```python
from build123d import *

# Parameters (mm, degrees)
SKETCH1_R          = 2.6924
EXTRUDE3_DEPTH     = 1.2446
SKETCH4_W          = 15.875
SKETCH4_H          = 1.4224
CHAMFER1_SIZE      = 0.47625
SKETCH26_R         = 0.7112
EXTRUDE8_DEPTH     = 1.2446
CUT_EXTRUDE3_REACH = 18.325
CIRPATTERN1_COUNT  = 4
DRAFT2_ANGLE       = 5


# Read off the part's stored shape, not the designer's step: Extrude10, Draft1
with BuildPart() as part:
    # Sketch1 → Extrude3 (new body)
    with BuildSketch(Plane.XY):
        Circle(SKETCH1_R)
    extrude(amount=EXTRUDE3_DEPTH)

    # Sketch11 → Cut-Revolve3 (revolve, cut)
    with BuildSketch(Plane(origin=(0, 0, 0), x_dir=(0, 0, -1), z_dir=(1, 0, 0)), mode=Mode.PRIVATE) as cut_revolve3_sk:
        Polygon((0, 1.209143479), (-1.2446, 2.6924), (0, 2.6924), align=None)
    revolve(cut_revolve3_sk.sketch.rotate(Axis((0, 0, -0.441444004), (0, 0, 1)), 90), axis=Axis((0, 0, -0.441444004), (0, 0, 1)), mode=Mode.SUBTRACT)

    # Extrude10 outline → Extrude10 (revolve)
    with BuildSketch(Plane.XZ):
        Polygon((1.4224, 0), (1.4224, 0.178943468), (1.209143479, 0.178943468), (1.209143479, 0), (0, 0), (0, -1.4224), align=None)
    revolve(axis=Axis((0, 0, 0), (0, 0, 1)))



with BuildPart() as body_2:
    # Sketch4 → Revolve1 (revolve)
    with BuildSketch(Plane(origin=(0, 0, 0), x_dir=(0, 0, -1), z_dir=(1, 0, 0)), mode=Mode.PRIVATE) as revolve1_sk:
        with Locations((6.6929, 0.7112)):
            Rectangle(SKETCH4_W, SKETCH4_H)
    revolve(revolve1_sk.sketch.rotate(Axis((0, 0, 1.2446), (0, 0, -1)), 180), axis=Axis((0, 0, 1.2446), (0, 0, -1)))

    # Chamfer1
    chamfer1_edges = [body_2.edges().sort_by_distance(p)[0] for p in [
        (0, 1.4224, -14.6304),
    ]]
    chamfer(chamfer1_edges, length=CHAMFER1_SIZE)


with BuildPart() as part_1:
    add(part.part)

    add(body_2.part)  # Extrude8 merges body 2
    # Sketch26 → Extrude8 (add)
    with BuildSketch(Plane.XY.offset(1.2446)):
        Circle(SKETCH26_R)
    extrude(amount=-EXTRUDE8_DEPTH)

    # Cut-Extrude3: up to this cone (the profile starts inside it)
    cut_extrude3_end = Plane(origin=(0, 0, 1.2446), z_dir=(0, 0, 1)).offset(-1.673411083) * Cone(1.192e-06, 26.805764308, 22.492705944, align=(Align.CENTER, Align.CENTER, Align.MIN), mode=Mode.PRIVATE)
    # Sketch12 → Cut-Extrude3 (cut, up to the surface)
    with BuildSketch(Plane.XY.offset(1.2446), mode=Mode.PRIVATE) as cut_extrude3_sk1:
        with BuildLine():
            Line((1.758668316, 0.358986667), (1.058827491, 0.358986667))
            Line((1.058827491, 0.358986667), (0.563965298, 0.563965298))
            Line((0.563965298, 0.563965298), (0.358986667, 1.058827491))
            Line((0.358986667, 1.058827491), (0.358986667, 1.758668316))
            ThreePointArc((0.358986667, 1.758668316), (0.180406886, 1.785844066), (0, 1.794933333))
            Line((0, 1.794933333), (0, 0))
            Line((0, 0), (1.794933333, 0))
            ThreePointArc((1.794933333, 0), (1.785844066, 0.180406886), (1.758668316, 0.358986667))
        make_face()
    cut_extrude3_tool1 = extrude(cut_extrude3_sk1.sketch, amount=-CUT_EXTRUDE3_REACH, mode=Mode.PRIVATE) & cut_extrude3_end
    cut_extrude3 = cut_extrude3_tool1.solids().sort_by_distance((1.408748, 0.333602, 1.2446))[0]
    add(cut_extrude3, mode=Mode.SUBTRACT)

    # CirPattern1: Cut-Extrude3 ×4 about axis
    cirpattern1_axis = Axis((0, 0, 0), (0, 0, 1))
    for i in range(1, CIRPATTERN1_COUNT):
        add(cut_extrude3.rotate(cirpattern1_axis, i * 360 / CIRPATTERN1_COUNT), mode=Mode.SUBTRACT)

    # Draft1 outline → Draft1 (revolve)
    with BuildSketch(Plane.XZ):
        Polygon((1.794933333, 1.2446), (1.737108581, 1.028795087), (1.794933333, 1.028795087), align=None)
    revolve(axis=Axis((0, 0, 0), (0, 0, 1)))

    # Draft2
    draft2_faces = [part_1.faces().sort_by_distance(p)[0] for p in [
        (0.358986667, 1.329150829, 0.986428177),
        (0.466729534, 0.798713199, 0.799402029),
        (0.798713199, 0.466729534, 0.799402029),
        (1.329150829, 0.358986667, 0.986428177),
        (1.329150829, -0.358986667, 0.986428177),
        (0.798713199, -0.466729534, 0.799402029),
        (0.466729534, -0.798713199, 0.799402029),
        (0.358986667, -1.329150829, 0.986428177),
        (-0.358986667, -1.329150829, 0.986428177),
        (-0.466729534, -0.798713199, 0.799402029),
        (-0.798713199, -0.466729534, 0.799402029),
        (-1.329150829, -0.358986667, 0.986428177),
        (-1.329150829, 0.358986667, 0.986428177),
        (-0.798713199, 0.466729534, 0.799402029),
        (-0.466729534, 0.798713199, 0.799402029),
        (-0.358986667, 1.329150829, 0.986428177),
    ]]
    draft(draft2_faces, Plane(origin=(0, 1.4224, 1.2446), x_dir=(0, 1, 0), z_dir=(0, 0, 1)), DRAFT2_ANGLE)


solid = part_1.part
```
Geometry: final body of the model. Coordinates: model frame, mm. Coordinates: 2 decimals unless noted, no trailing zeros. Order: outer loops, then holes, each group sorted by start corner. A loop starts at its lowest first (then second) coordinate and runs counter-clockwise, first axis right, second up.
Item 1: Section query A-A (z = -13.5). Output: boundary loops of the cut face in (x, y), then the cut area to 3 significant figures.
Answer:
outline: circle Ø2.84 at (0, 0)
area: 6.36 mm2
Item 2: Material intervals for line 1 along Y through (x, z) = (-0.1, -3.25); line 2 along Z through (x, y) = (0.25, 1); line 3 along X through (y, z) = (0.85, -5.75), sorted ascending.
Answer:
line 1: y = -1.42 to 1.42
line 2: z = -14.55 to 0.44
line 3: x = -1.14 to 1.14
Item 3: Contact query for flat-ended pins moving along their axis: P1, Ø1.5, axis at x = 0.5, z = -6.5, coming from the +Y side; P2, Ø3, axis at y = 1, z = -10, coming from the -X side; P3, Ø2, axis at x = 1, y = 1.5, coming from the -Z side. Output: stop coordinate, or through.
Answer:
P1: stops at y = 1.42
P2: stops at x = -1.42
P3: stops at z = -14.63
Item 4: Draft query along X for faces 1 (the face through (0, 0, -14.63)), 2 (the face through (0.013, 0.301, -0.176)). Return one class per face: released by +X, released by -X, zero draft, split by the parting line, or undercut.
Answer:
face 1: zero draft
face 2: undercut
